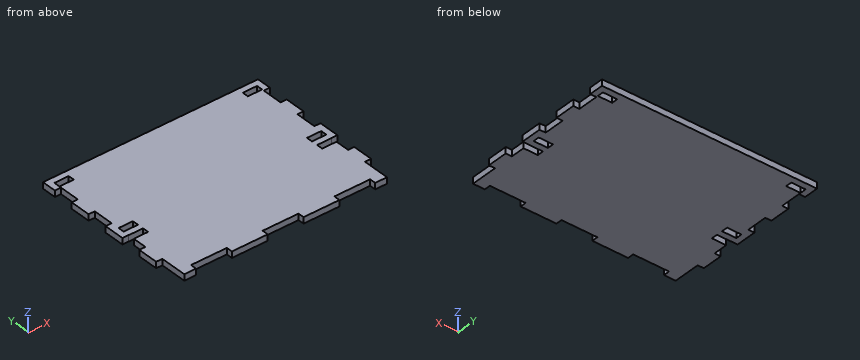
Autodesk Inventor part; units mm, degrees
ref_plane "YZ Plane" through (0, 0, 0) normal (1, 0, 0) x (0, 1, 0)
ref_plane "XZ Plane" through (0, 0, 0) normal (0, 1, 0) x (-1, 0, 0)
ref_plane "XY Plane" through (0, 0, 0) normal (0, 0, 1) x (1, 0, 0)
sketch "Sketch1" plane through (0, 0, 0) normal (0, 0, 1) x (1, 0, 0)
  line L0 (0, 0) -> (99, 0)
  line L1 (99, 0) -> (99, 77)
  line L2 (99, 77) -> (0, 77)
  line L3 (0, 77) -> (0, 0)
  dimension "d0" = 99
  dimension "d1" = 77
extrude "Extrusion1" add sketch "Sketch1" along normal blind 3
sketch "Sketch2" plane through (0, 0, 3) normal (0, 0, 1) x (1, 0, 0)
  line L0 (99, 77) -> (0, 77)
  line L1 (0, 0) -> (99, 0)
  line L2 (0, 77) -> (99, 77)
  line L3 (99, 77) -> (99, 0)
  line L4 (99, 0) -> (0, 0)
  line L5 (0, 0) -> (0, 77)
  line L6 (0, 77) -> (0, 0)
  line L7 (0, 10) -> (-3, 10)
  line L8 (-3, 10) -> (-3, 20)
  line L9 (-3, 20) -> (0, 20)
  line L10 (-3, 40) -> (0, 40)
  line L11 (-3, 30) -> (-3, 40)
  line L12 (0, 30) -> (-3, 30)
  line L13 (-3, 60) -> (0, 60)
  line L14 (-3, 50) -> (-3, 60)
  line L15 (0, 50) -> (-3, 50)
  line L16 (99, 77) -> (0, 77)
  line L17 (0, 77) -> (-3, 77)
  line L18 (-3, 77) -> (-3, 70)
  line L19 (-3, 70) -> (0, 70)
  line L20 (99, 0) -> (99, 77)
  line L21 (99, 77) -> (102, 77)
  line L22 (102, 77) -> (102, 70)
  line L23 (102, 70) -> (99, 70)
  line L24 (99, 0) -> (99, 77)
  line L25 (99, 60) -> (102, 60)
  line L26 (102, 60) -> (102, 50)
  line L27 (102, 50) -> (99, 50)
  line L28 (99, 40) -> (102, 40)
  line L29 (102, 40) -> (102, 30)
  line L30 (102, 30) -> (99, 30)
  line L31 (99, 20) -> (102, 20)
  line L32 (102, 20) -> (102, 10)
  line L33 (102, 10) -> (99, 10)
  line L34 (99, 10) -> (99, -3)
  line L35 (99, -3) -> (93.25, -3)
  line L36 (93.25, -3) -> (93.25, 0)
  line L37 (93.25, 0) -> (75.75, 0)
  line L38 (75.75, 0) -> (75.75, -3)
  line L39 (75.75, -3) -> (58.25, -3)
  line L40 (58.25, -3) -> (58.25, 0)
  line L41 (58.25, 0) -> (40.75, 0)
  line L42 (40.75, 0) -> (40.75, -3)
  line L43 (40.75, -3) -> (23.25, -3)
  line L44 (23.25, -3) -> (23.25, 0)
  line L45 (23.25, 0) -> (5.75, 0)
  line L46 (5.75, 0) -> (5.75, -3)
  line L47 (5.75, -3) -> (0, -3)
  line L48 (0, -3) -> (0, 0)
  point P0 (99, 30)
  point P1 (99, 20)
  point P2 (99, 10)
  point P3 (23.25, 0)
  point P4 (58.25, 0)
  point P5 (93.25, 0)
  dimension "d13" = 3
  dimension "d14" = 10
  dimension "d17" = 20
  dimension "d22" = 3
  dimension "d23" = 7
  dimension "d24" = 3
  dimension "d48" = 13
  dimension "d49" = 5.75
  dimension "d50" = 17.5
  dimension "d51" = 17.5
  dimension "d52" = 17.5
  dimension "d53" = 17.5
  dimension "d54" = 17.5
  dimension "d55" = 5.75
extrude "Extrusion2" add sketch "Sketch2" against normal blind 3 contours L21 L22 L23 L3 | L5 L19 L18 L17 | L25 L26 L27 L3 | L5 L15 L14 L13 | L28 L29 L30 L3 | L5 L12 L11 L10 | L31 L32 L33 L3 | L5 L7 L8 L9 | L34 L35 L36 L1 | L1 L46 L47 L48 | L38 L39 L40 L1 | L1 L42 L43 L44
sketch "Sketch3" plane through (0, 0, 3) normal (0, 0, 1) x (1, 0, 0)
  line L0 (0, 73.9) -> (7, 73.9)
  line L1 (7, 73.9) -> (7, 70.9)
  line L2 (7, 70.9) -> (0, 70.9)
  line L3 (0, 70.9) -> (0, 73.9)
  line L4 (92, 73.9) -> (99, 73.9)
  line L5 (99, 73.9) -> (99, 70.9)
  line L6 (99, 70.9) -> (92, 70.9)
  line L7 (92, 70.9) -> (92, 73.9)
  line L8 (0, 35.9) -> (7, 35.9)
  line L9 (7, 35.9) -> (7, 32.9)
  line L10 (7, 32.9) -> (0, 32.9)
  line L11 (0, 32.9) -> (0, 35.9)
  line L12 (92, 35.9) -> (99, 35.9)
  line L13 (99, 35.9) -> (99, 32.9)
  line L14 (99, 32.9) -> (92, 32.9)
  line L15 (92, 32.9) -> (92, 35.9)
  line L16 (7, 29.9) -> (7, 26.9)
  line L17 (7, 26.9) -> (0, 26.9)
  line L18 (0, 26.9) -> (0, 29.9)
  line L19 (0, 29.9) -> (7, 29.9)
  line L20 (99, 35.9) -> (99, 32.9)
  line L21 (99, 32.9) -> (92, 32.9)
  line L22 (92, 32.9) -> (92, 35.9)
  line L23 (92, 35.9) -> (99, 35.9)
  line L24 (99, 29.9) -> (99, 26.9)
  line L25 (99, 26.9) -> (92, 26.9)
  line L26 (92, 26.9) -> (92, 29.9)
  line L27 (92, 29.9) -> (99, 29.9)
  line L28 (-3, 77) -> (102, 77)
  line L29 (99, 20) -> (99, 30)
  point P0 (0, 0)
  dimension "d27" = 7
  dimension "d28" = 3
  dimension "d31" = 92
  dimension "d34" = 38
  dimension "d41" = 6
  dimension "d44" = 92
  dimension "d47" = 3.1
extrude "Extrusion3" cut sketch "Sketch3" against normal through all
properties part number "DoosjeVoorkant" material "Wood (Cherry)"
Geometry check sheet. Reference: the model listing, model coordinates, mm. Round coordinates to 2 decimals unless told otherwise and drop trailing zeros. Write each loop counter-clockwise with the first axis right and the second up, starting at its lowest first coordinate (ties: lowest second). Pieces come first, ordered by that corner, then holes. Notation, with made-up numbers: (15, -1.75) -> (67, -1.75) arc R21 cw to (67, 35.25) -> close; hole circle Ø7 at (39, -15.5). An arc over 180 degrees is marked (long way). Put each result on its own line as item: value.
1) Cross-section at B-B, the plane y = 43.5. Enter the section's corners in (x, z), plus the area to 3 significant figures.
Recorded:
outline: (0, 0) -> (99, 0) -> (99, 3) -> (0, 3) -> close
area: 297 mm2
2) Thickness scan on probe 1 along Y at (x, z) = (97, 1.95); probe 2 along X at (y, z) = (34, 1.9); probe 3 along X at (y, z) = (4, 2.2). Record the ranges inside material, lowest first. Write a range as from..to.
Recorded:
probe 1: y = -3..26.9, 29.9..32.9, 35.9..70.9, 73.9..77
probe 2: x = -3..0, 7..92, 99..102
probe 3: x = 0..99
3) Cross-section at C-C, the plane x = 14.5. Enter the section's corners in (y, z).
Recorded:
outline: (0, 0) -> (77, 0) -> (77, 3) -> (0, 3) -> close
4) Depth check by flat-ended pin: P1, Ø1.5, axis at x = -2, z = 1, coming from the -Y side; P2, Ø0.9, axis at x = 82, z = 2, coming from the -Y side. Enter the tip coordinate at first touch or a pass-through.
Recorded:
P1: stops at y = 10
P2: stops at y = 0
5) Cross-section at A-A, the plane z = 0.6. Give the number of separate pieces and of enclosed holes in the cut face, plus the area to 3 significant figures.
Recorded:
separate pieces: 1
enclosed holes: 4
area: 7,860 mm2
